Can you work these out from the model? Positions are in its coordinate system, mm. Face numbers are marked on the shaded views. A direction names the side the tool comes from. Round coordinates to 2 decimals unless told otherwise and drop trailing zeros. Loops run counter-clockwise (first coordinate to the right, second up) from the corner with the lowest first, then second, coordinate; pieces in that order, holes last.
(1) Will these pins go through, and if not, where does the flat tip stop? pin 1 Ø7.5 at (x, y) = (8, 1) entering from +Z; pin 2 Ø2 at (x, z) = (3, 7) entering from +Y.
(2) I want a section at C-C on x = 3. Write out the boundary of the cut face in (y, z) (3 decimals), plus the area to 3 significant figures.
(3) Thinking about a two-plate mould opening in Y: for the marked faces 4, 5 and 6, which applies, released by +Y, released by -Y, zero draft, split by the parting line, or undercut?
(4) Which directions (+Z, -Z, +X, -X, +Y, -Y) give clear straight access to the entire face, cutting with the end or side of a thin tool? Please do the marked faces 1, 2 and 3.
(5) I want a section at A-A on z = 3.5. Write out the boundary of the cut face in (x, y), plus the area to 3 significant figures.
(6) I want a section at B-B on y = 23. Write out the boundary of the cut face in (x, z) (3 decimals), plus the area to 3 significant figures.
(7) If I drill on line 1 along Z through (x, y) = (3, 23.35) (3 decimals); line 2 along Y through (x, z) = (1.25, 6); line 3 along Z through (x, y) = (12, 21), over which ranges is the centre line in solid material (lowest first)?
(8) I want a section at D-D on x = 7.5. Write out the boundary of the cut face in (y, z) (3 decimals), plus the area to 3 significant figures.
from build123d import *

# Parameters (mm, degrees)
F0_W     = 30
F0_H     = 5
F1_DEPTH = 15
F3_R     = 1.775
F4_DEPTH = 25
F2_R     = 1.775
F2_R_2   = 1.75
F5_DEPTH = 25


with BuildPart() as f1:
    # F0 (on Right) → F1 (new body)
    with BuildSketch(Plane.YZ):
        Polygon((-8.125334, 10), (-13.998746, 10), (-13.998746, -10), (-8.125334, -10), (-8.125334, -2.5), (-8.125334, 2.5), align=None)
        with Locations((6.874666, 0)):
            Rectangle(F0_W, F0_H)
        Polygon((21.874666, 10), (21.874666, 2.5), (21.874666, -2.5), (21.874666, -10), (26.874666, -10), (26.874666, 10), align=None)
    extrude(amount=F1_DEPTH)

    # F3 (on face) → F4 (cut)
    with BuildSketch(Plane(origin=(0, -8.125334, 0), x_dir=(-1, 0, 0), z_dir=(0, 1, 0))):
        with Locations((-7.5, 6.25)):
            Circle(F3_R)
    extrude(amount=-F4_DEPTH, mode=Mode.SUBTRACT)

    # F2 (on face) → F5 (cut)
    with BuildSketch(Plane(origin=(0, 26.874666, 0), x_dir=(-1, 0, 0), z_dir=(0, 1, 0))):
        with Locations((-12, 7)):
            Circle(F2_R)
        with Locations((-3, 7)):
            Circle(F2_R)
        with Locations((-3, -7)):
            Circle(F2_R)
        with Locations((-12, -7)):
            Circle(F2_R_2)
    extrude(amount=-F5_DEPTH, mode=Mode.SUBTRACT)


solid = f1.part
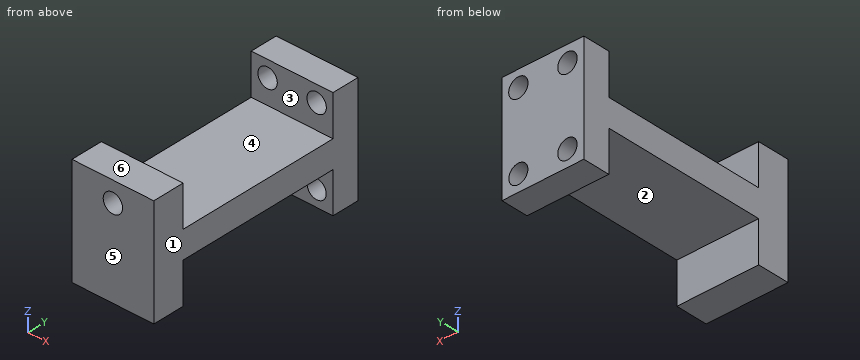
Filled sheet:
1. pin 1: stops at z = 2.5
1. pin 2: stops at y = -8.13
2. outline: (-13.999, -10) - (-8.125, -10) - (-8.125, -2.5) - (21.875, -2.5) - (21.875, -5.225) - (26.875, -5.225) - (26.875, 5.225) - (21.875, 5.225) - (21.875, 2.5) - (-8.125, 2.5) - (-8.125, 10) - (-13.999, 10) - close; (21.875, -10) - (26.875, -10) - (26.875, -8.775) - (21.875, -8.775) - close; (21.875, 8.775) - (26.875, 8.775) - (26.875, 10) - (21.875, 10) - close
2. area: 332 mm2
3. face 4: undercut
3. face 5: released by -Y
3. face 6: zero draft
4. face 1: +Z, -Z, +X, +Y, -Y
4. face 2: -Z, +X, -X
4. face 3: +Z, +X, -X
5. outline: (0, -14) - (15, -14) - (15, -8.13) - (0, -8.13) - close; (0, 21.87) - (15, 21.87) - (15, 26.87) - (0, 26.87) - close
5. area: 163 mm2
6. outline: (0, -10) - (15, -10) - (15, 10) - (0, 10) - close; hole circle Ø3.55 at (3, -7); hole circle Ø3.55 at (3, 7); hole circle Ø3.55 at (12, 7); hole circle Ø3.5 at (12, -7)
6. area: 261 mm2
7. line 1: z = -10 to -8.775, -5.225 to 5.225, 8.775 to 10
7. line 2: y = -14 to -8.13, 21.87 to 26.87
7. line 3: z = -2.5 to 2.5
8. outline: (-13.999, -10) - (-8.125, -10) - (-8.125, -2.5) - (21.875, -2.5) - (21.875, -10) - (26.875, -10) - (26.875, 10) - (21.875, 10) - (21.875, 2.5) - (-8.125, 2.5) - (-8.125, 4.475) - (-13.999, 4.475) - close; (-13.999, 8.025) - (-8.125, 8.025) - (-8.125, 10) - (-13.999, 10) - close
8. area: 347 mm2
